For this review, use the dimensioned drawing (mm, ordinates from the lowest corner) and the shaded views. A direction names the side the tool comes from. Coordinates: 2 decimals unless noted, no trailing zeros. Write each loop counter-clockwise with the first axis right and the second up, starting at its lowest first coordinate (ties: lowest second). Pieces come first, ordered by that corner, then holes.
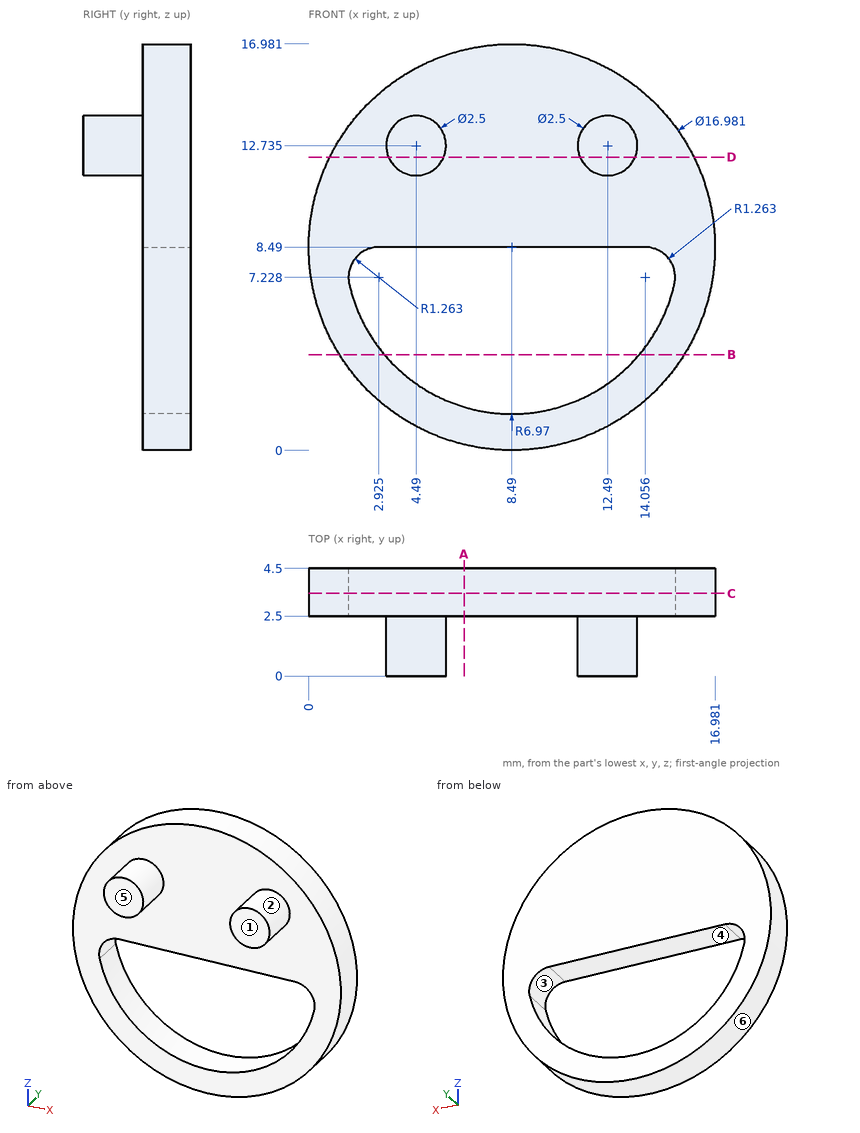
Item 1: Machinability: for the marked faces 1, 2 and 3, which of the approach directions +Z, -Z, +X, -X, +Y, -Y give a long, thin tool a straight path to every point of the face, cutting with its end or side? Answer none if there is none.
Solved:
face 1: +Z, -Z, +X, -X, -Y
face 2: -Y
face 3: +Y, -Y
Item 2: Take a section at A-A, the plane x = 6.5. Write out the cut boundary in (y, z).
Solved:
outline: (2.5, 0.24) - (4.5, 0.24) - (4.5, 1.81) - (2.5, 1.81) - close; (2.5, 8.49) - (4.5, 8.49) - (4.5, 16.74) - (2.5, 16.74) - close
Item 3: Mouldability with a two-part tool opening along X and no side actions: class the marked faces 4, 5 and 6 as pulls with the +X half, pulls with the -X half, needs draft (parallel to the pull), parting line crosses it, or undercut.
Solved:
face 4: undercut
face 5: needs draft
face 6: parting line crosses it
Item 4: Take a section at B-B, the plane z = 4. Write out the cut boundary in (x, y) (1 decimal).
Solved:
outline: (1.3, 2.5) - (3.2, 2.5) - (3.2, 4.5) - (1.3, 4.5) - close; (13.8, 2.5) - (15.7, 2.5) - (15.7, 4.5) - (13.8, 4.5) - close
Item 5: Take a section at C-C, the plane y = 3.45. Write out the cut boundary in (x, z) (1 decimal).
Solved:
outline: circle Ø17 at (8.5, 8.5); hole (1.7, 6.9) arc R7 ccw to (15.3, 6.9) arc R1.3 ccw to (14.1, 8.5) - (2.9, 8.5) arc R1.3 ccw to start
Item 6: For pin 1 (2 mm diameter, centred on y = 4, z = 12, fed in from +X); pin 2 (1.5 mm diameter, centred on y = 3, z = 13, fed in from -X); pin 3 (1.5 mm diameter, centred on x = 14.5, y = 3, fed in from -Z) (1 decimal), all flat-tipped, find the tip position at first contact; note any pin that passes through.
Solved:
pin 1: stops at x = 16.6
pin 2: stops at x = 0.88
pin 3: stops at z = 1.8
Item 7: To check wall thickness, follow line 1 along Z through (x, y) = (4.5, 2.55) (1 decimal); line 2 along Y through (x, z) = (2.5, 4.5); line 3 along Z through (x, y) = (3, 3.15) (1 decimal). State the ranges of each line that lie inside material, in increasing order.
Solved:
line 1: z = 1 to 2.8, 8.5 to 16
line 2: y = 2.5 to 4.5
line 3: z = 2 to 4.2, 8.5 to 15
Item 8: Take a section at D-D, the plane z = 12.25. Write out the cut boundary in (x, y).
Solved:
outline: (0.88, 2.5) - (3.34, 2.5) - (3.34, 0) - (5.64, 0) - (5.64, 2.5) - (11.34, 2.5) - (11.34, 0) - (13.64, 0) - (13.64, 2.5) - (16.1, 2.5) - (16.1, 4.5) - (0.88, 4.5) - close
